Read the model definition and answer for the solid it produces. Units are mm, in the model's axes. A direction names the side the tool comes from. Round coordinates to 2 decimals unless told otherwise and drop trailing zeros. Write each loop counter-clockwise with the first axis right and the second up, starting at its lowest first coordinate (ties: lowest second). Pieces come first, ordered by that corner, then holes. Notation, with made-up numbers: (-10, 20) - (3, 20) arc R24 ccw to (3, 43) - close; hole circle Ø10 at (-12, -10). An arc over 180 degrees is marked (long way). Answer as CSV lines item,"result". Start each with the question number.
1) Find section A-A on z = 3.5. State how many separate pieces and enclosed holes the cut face has, then the cut area to 3 significant figures.
2) Consider line 1 along X through (y, z) = (26.25, 10); line 2 along Y through (x, z) = (26, 3); line 3 along X through (y, z) = (30.5, 9). Determine where each line is inside the solid, lowest interval first.
3) Find section D-D on x = 50.5. Determine the outline of the cut face in (y, z).
4) Find section B-B on y = 22. Determine the outline of the cut face in (x, z), then the cut area to 4 significant figures.
5) Which of the six approach directions +Z, -Z, +X, -X, +Y, -Y give full straight-line access (tool end or side, diameter ignored) to faces 5 (the flat face through (38, 39.879, 6)), 6 (the flat face through (21.48, 32, 6)), 7 (the flat face through (26, 23.329, 6))?
6) This flat-tipped pin is pushed along its axis until it touches: pin 1 (1 mm diameter, centred on x = 45.5, z = 7.5, fed in from -Y). Where does it stop, or does it pass through?
7) Find section C-C on x = 41.5. Determine the outline of the cut face in (y, z), then the cut area to 3 significant figures.
8) For a pull along Y with two mould halves and no side action, classify faces 1 (the flat face through (22.5, 42.9, 5.9)), 2 (the flat face through (26, 18.879, 6)), 3 (the flat face through (23.93, 25, 6)), 4 (the flat face through (77.605, 31, 6)) as +Y half, -Y half, draft (parallel to the pull), parting line (faces both ways), or undercut.
from build123d import *

# Parameters (mm, degrees)
ESBO_O2_W                = 2.5
ESBO_O2_H                = 2.5
RESSALTO_EXTRUS_O1_DEPTH = 12
ESBO_O5_W                = 0.7
ESBO_O5_H                = 2.5
RESSALTO_EXTRUS_O2_DEPTH = 12
ESBO_O7_W                = 3.1
ESBO_O7_H                = 3.1
CORTE_EXTRUS_O5_DEPTH    = 90.954849667


with BuildPart() as part:
    # Esboço2 → Ressalto-extrusão1 (new body)
    with BuildSketch(Plane.XY):
        Polygon((70.72996521, 18.87874794), (75.60496521, 18.87874794), (77.60496521, 20.87874794), (77.60496521, 41.878746033), (75.60496521, 43.878746033), (23.479967117, 43.878746033), (21.479967117, 41.878746033), (21.479967117, 20.87874794), (23.479967117, 18.87874794), (28.229967117, 18.87874794), (28.229967117, 38.878746033), (29.229967117, 39.878746033), (46.47996521, 39.878746033), (46.47996521, 42.378746033), (53.47996521, 42.378746033), (60.47996521, 42.378746033), (60.47996521, 39.878746033), (69.72996521, 39.878746033), (70.72996521, 38.878746033), align=None)
        with Locations((25.479967117, 34.878746033)):
            Rectangle(ESBO_O2_W, ESBO_O2_H, mode=Mode.SUBTRACT)
        with Locations((25.479967117, 24.87874794)):
            Rectangle(ESBO_O2_W, ESBO_O2_H, mode=Mode.SUBTRACT)
        with Locations((73.47996521, 34.878746033)):
            Rectangle(ESBO_O2_W, ESBO_O2_H, mode=Mode.SUBTRACT)
        with Locations((73.47996521, 24.87874794)):
            Rectangle(ESBO_O2_W, ESBO_O2_H, mode=Mode.SUBTRACT)
    extrude(amount=RESSALTO_EXTRUS_O1_DEPTH)

    # Esboço5 → Ressalto-extrusão2 (add, through all)
    with BuildSketch(Plane(origin=(0, 0, 0), x_dir=(-1, 0, 0), z_dir=(0, 0, -1))):
        with Locations((-60.12996521, 41.128746033)):
            Rectangle(ESBO_O5_W, ESBO_O5_H)
        with Locations((-46.82996521, 41.128746033)):
            Rectangle(ESBO_O5_W, ESBO_O5_H)
    extrude(amount=-RESSALTO_EXTRUS_O2_DEPTH)

    # Esboço7 → Corte-extrusão5 (cut, through all)
    with BuildSketch(Plane(origin=(0, 0, 0), x_dir=(-1, 0, 0), z_dir=(0, 0, -1))):
        with Locations((-73.47996521, 34.878746033)):
            Rectangle(ESBO_O7_W, ESBO_O7_H)
        with Locations((-73.47996521, 24.87874794)):
            Rectangle(ESBO_O7_W, ESBO_O7_H)
        with Locations((-25.479967117, 24.87874794)):
            Rectangle(ESBO_O7_W, ESBO_O7_H)
        with Locations((-25.479967117, 34.878746033)):
            Rectangle(ESBO_O7_W, ESBO_O7_H)
    extrude(amount=-CORTE_EXTRUS_O5_DEPTH, mode=Mode.SUBTRACT)


solid = part.part
Check values:
1,separate pieces,"1"
1,enclosed holes,"4"
1,area,"434 mm^2"
2,line 1,"x = 21.48 to 23.93, 27.03 to 28.23, 70.73 to 71.93, 75.03 to 77.6"
2,line 2,"y = 18.88 to 23.33, 26.43 to 33.33, 36.43 to 43.88"
2,line 3,"x = 21.48 to 28.23, 70.73 to 77.6"
3,outline,"(42.38, 0) - (43.88, 0) - (43.88, 12) - (42.38, 12) - close"
4,outline,"(21.48, 0) - (28.23, 0) - (28.23, 12) - (21.48, 12) - close; (70.73, 0) - (77.6, 0) - (77.6, 12) - (70.73, 12) - close"
4,area,"163.5 mm^2"
5,face 5,"+Z, -Z, -Y"
5,face 6,"+Z, -Z, -X, +Y, -Y"
5,face 7,"+Z, -Z"
6,pin 1,"stops at y = 39.88"
7,outline,"(39.88, 0) - (43.88, 0) - (43.88, 12) - (39.88, 12) - close"
7,area,"48.0 mm^2"
8,face 1,"+Y half"
8,face 2,"-Y half"
8,face 3,"undercut"
8,face 4,"draft"
